```python
from build123d import *

# Parameters (mm, degrees)
F1_DEPTH = 3.175


with BuildPart() as f1:
    # F0 (on Front) → F1 (new body)
    with BuildSketch(Plane.XZ):
        Polygon((98.386274, 16.736827), (-51.613726, 16.736827), (-99.901127, 16.736827), (-99.901127, -43.263173), (-51.613726, -43.263173), (98.386274, -43.263173), (256.824182, -43.263173), (256.824182, 16.736827), align=None)
        with BuildLine():
            Line((-16.563727, -10.134648), (-16.563727, -6.324648))
            ThreePointArc((-16.563727, -6.324648), (-8.906867, -9.311239), (-0.751226, -10.327486))
            ThreePointArc((-0.751226, -10.327486), (7.404414, -9.311239), (15.061274, -6.324648))
            Line((15.061274, -6.324648), (15.061274, -10.134648))
            ThreePointArc((15.061274, -10.134648), (7.404414, -13.121239), (-0.751226, -14.137486))
            ThreePointArc((-0.751226, -14.137486), (-8.906867, -13.121239), (-16.563727, -10.134648))
        make_face(mode=Mode.SUBTRACT)
        with BuildLine():
            Line((142.061274, -10.134648), (142.061274, -6.324648))
            ThreePointArc((142.061274, -6.324648), (157.788284, -10.327282), (173.486782, -6.214243))
            Line((173.486782, -6.214243), (173.486782, -10.024243))
            ThreePointArc((173.486782, -10.024243), (157.788284, -14.137275), (142.061274, -10.134648))
        make_face(mode=Mode.SUBTRACT)
    extrude(amount=F1_DEPTH)


solid = f1.part
```
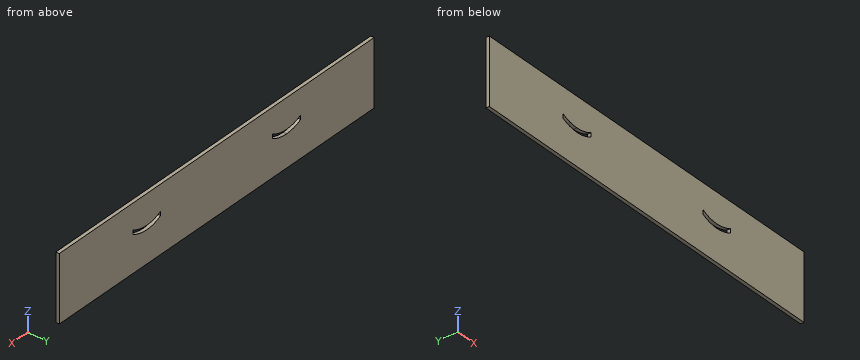
The listing builds one solid part. Answer for the finished solid, in the listing's coordinates (mm). Give positions to 0.01 mm unless a question says otherwise; leave off trailing zeros. Order: outer loops, then holes, each group sorted by start corner. A loop starts at its lowest first (then second) coordinate and runs counter-clockwise, first axis right, second up.
Item 1: The part is cut by section A-A, the plane x = 157.5. Give the vertices of the cut face in (y, z) (3 decimals), and give its area (3 significant figures).
From the geometry:
outline: (-3.175, -43.263) - (0, -43.263) - (0, -14.137) - (-3.175, -14.137) - close; (-3.175, -10.327) - (0, -10.327) - (0, 16.737) - (-3.175, 16.737) - close
area: 178 mm2
Item 2: Given pin 1 Ø1 at (x, z) = (165, -6.5) entering from +Y, flat-ended and moving along its own axis, determine where the tip first touches the part or whether it passes through.
From the geometry:
pin 1: stops at y = 0
Item 3: Find the intervals of material crossed by probe 1 along Z at (x, y) = (156, -2.15); probe 2 along X at (y, z) = (-0.45, -7.5); probe 3 along Z at (x, y) = (171.5, -2.75), in increasing order.
From the geometry:
probe 1: z = -43.26 to -14.09, -10.28 to 16.74
probe 2: x = -99.9 to -16.56, -14.17 to 12.66, 15.06 to 142.06, 144.43 to 170.92, 173.49 to 256.82
probe 3: z = -43.26 to -11.04, -7.23 to 16.74
